Read the model definition and answer for the solid it produces. Units are mm, in the model's axes. A direction names the side the tool comes from. Coordinates: 2 decimals unless noted, no trailing zeros. Loops run counter-clockwise (first coordinate to the right, second up) from the corner with the lowest first, then second, coordinate; pieces in that order, holes last. Notation, with made-up numbers: (54.5, 63) -> (106.5, 63) arc R35 ccw to (106.5, 96) -> close; hole circle Ø10 at (1, -23). An arc over 180 degrees is marked (long way). Answer as a JSON object with one key per item and string values. Group by question number.
Q1. For faces 5 (the flat face through (-36.31, 0.99, 31.46)), 6 (the flat face through (36.307, 0.986, -31.462)), 7 (the flat face through (25.97, 0.99, -40.41)), determine the directions among +Z, -Z, +X, -X, +Y, -Y from which every point of the face is accessible in a straight line to the end or side of a thin tool.
Q2. The part is cut by section B-B on x = 29.5. Write down the section's boundary in (y, z).
Q3. Determine the mould class of faces 1 (the flat face through (36.307, 0.986, 31.462)), 2 (the flat face through (43.701, 0.986, 19.956)), 3 (the cylindrical face through (37.81, 0.99, 24.4)), 4 (the flat face through (43.701, 0.986, -19.956)) for opening direction Z: released by +Z, released by -Z, zero draft, split by the parting line, or undercut.
Q4. This flat-tipped pin is pushed along its axis until it touches: P1, Ø5, axis at x = 10.5, z = -1.5, coming from the -Y side. Where does it stop, or does it pass through?
Q5. The part is cut by section C-C on z = -26. Write down the section's boundary in (x, y).
Q6. Straight lines are drawn through the part: line 1 along Z through (x, y) = (-27, 0.9); line 2 along X through (y, z) = (0.65, 0); line 3 along Z through (x, y) = (5, 0.85). For each, find the intervals that lie inside material, in ascending order. Write a range as [from, to].
Q7. The part is cut by section A-A on z = -3. Write down the section's boundary in (x, y).
from build123d import *

# Parameters (mm, degrees)
SKETCH1_R                 = 45
BOSS_EXTRUDE1_DEPTH       = 2
BOSS_EXTRUDE2_DEPTH       = 2
CIRPATTERN1_COUNT         = 11
CIRPATTERN1_COPY_1_DEPTH  = 2
CIRPATTERN1_COPY_2_DEPTH  = 2
CIRPATTERN1_COPY_3_DEPTH  = 2
CIRPATTERN1_COPY_4_DEPTH  = 2
CIRPATTERN1_COPY_5_DEPTH  = 2
CIRPATTERN1_COPY_6_DEPTH  = 2
CIRPATTERN1_COPY_7_DEPTH  = 2
CIRPATTERN1_COPY_8_DEPTH  = 2
CIRPATTERN1_COPY_9_DEPTH  = 2
CIRPATTERN1_COPY_10_DEPTH = 2
SKETCH3_R                 = 12.5
CUT_EXTRUDE1_DEPTH        = 2


with BuildPart() as part:
    # Sketch1 → Boss-Extrude1 (new body)
    with BuildSketch(Plane(origin=(0, 0, 0), x_dir=(1, 0, 0), z_dir=(0, 1, 0))):
        Circle(SKETCH1_R)
    extrude(amount=BOSS_EXTRUDE1_DEPTH)

    # Sketch2 → Boss-Extrude2 (add)
    with BuildSketch(Plane(origin=(0, 0, 0), x_dir=(1, 0, 0), z_dir=(0, 1, 0))):
        with BuildLine():
            Line((0, 0), (-51, 0))
            ThreePointArc((-51, 0), (-50.870115566, -3.637491206), (-50.481123832, -7.256454825))
            Line((-50.481123832, -7.256454825), (0, 0))
        make_face()
    boss_extrude2 = extrude(amount=BOSS_EXTRUDE2_DEPTH)

    # Mirror1: Boss-Extrude2 across plane
    add(boss_extrude2.mirror(Plane.XY))

    # CirPattern1: Boss-Extrude2 ×11 about axis
    cirpattern1_axis = Axis((0, 0, 0), (0, 1, 0))
    for i in range(1, CIRPATTERN1_COUNT):
        add(boss_extrude2.rotate(cirpattern1_axis, i * 360 / CIRPATTERN1_COUNT))

    # CirPattern1 copy 1 sketch → CirPattern1 copy 1 (add)
    with BuildSketch(Plane(origin=(0, 0, 0), x_dir=(0.841253533, 0, -0.540640817), z_dir=(0, 1, 0))):
        with BuildLine():
            Line((0, 0), (-51, 0))
            ThreePointArc((-51, 0), (-50.870115566, 3.637491206), (-50.481123832, 7.256454825))
            Line((-50.481123832, 7.256454825), (0, 0))
        make_face()
    extrude(amount=CIRPATTERN1_COPY_1_DEPTH)

    # CirPattern1 copy 2 sketch → CirPattern1 copy 2 (add)
    with BuildSketch(Plane(origin=(0, 0, 0), x_dir=(0.415415013, 0, -0.909631995), z_dir=(0, 1, 0))):
        with BuildLine():
            Line((0, 0), (-51, 0))
            ThreePointArc((-51, 0), (-50.870115566, 3.637491206), (-50.481123832, 7.256454825))
            Line((-50.481123832, 7.256454825), (0, 0))
        make_face()
    extrude(amount=CIRPATTERN1_COPY_2_DEPTH)

    # CirPattern1 copy 3 sketch → CirPattern1 copy 3 (add)
    with BuildSketch(Plane(origin=(0, 0, 0), x_dir=(-0.142314838, 0, -0.989821442), z_dir=(0, 1, 0))):
        with BuildLine():
            Line((0, 0), (-51, 0))
            ThreePointArc((-51, 0), (-50.870115566, 3.637491206), (-50.481123832, 7.256454825))
            Line((-50.481123832, 7.256454825), (0, 0))
        make_face()
    extrude(amount=CIRPATTERN1_COPY_3_DEPTH)

    # CirPattern1 copy 4 sketch → CirPattern1 copy 4 (add)
    with BuildSketch(Plane(origin=(0, 0, 0), x_dir=(-0.654860734, 0, -0.755749574), z_dir=(0, 1, 0))):
        with BuildLine():
            Line((0, 0), (-51, 0))
            ThreePointArc((-51, 0), (-50.870115566, 3.637491206), (-50.481123832, 7.256454825))
            Line((-50.481123832, 7.256454825), (0, 0))
        make_face()
    extrude(amount=CIRPATTERN1_COPY_4_DEPTH)

    # CirPattern1 copy 5 sketch → CirPattern1 copy 5 (add)
    with BuildSketch(Plane(origin=(0, 0, 0), x_dir=(-0.959492974, 0, -0.281732557), z_dir=(0, 1, 0))):
        with BuildLine():
            Line((0, 0), (-51, 0))
            ThreePointArc((-51, 0), (-50.870115566, 3.637491206), (-50.481123832, 7.256454825))
            Line((-50.481123832, 7.256454825), (0, 0))
        make_face()
    extrude(amount=CIRPATTERN1_COPY_5_DEPTH)

    # CirPattern1 copy 6 sketch → CirPattern1 copy 6 (add)
    with BuildSketch(Plane(origin=(0, 0, 0), x_dir=(-0.959492974, 0, 0.281732557), z_dir=(0, 1, 0))):
        with BuildLine():
            Line((0, 0), (-51, 0))
            ThreePointArc((-51, 0), (-50.870115566, 3.637491206), (-50.481123832, 7.256454825))
            Line((-50.481123832, 7.256454825), (0, 0))
        make_face()
    extrude(amount=CIRPATTERN1_COPY_6_DEPTH)

    # CirPattern1 copy 7 sketch → CirPattern1 copy 7 (add)
    with BuildSketch(Plane(origin=(0, 0, 0), x_dir=(-0.654860734, 0, 0.755749574), z_dir=(0, 1, 0))):
        with BuildLine():
            Line((0, 0), (-51, 0))
            ThreePointArc((-51, 0), (-50.870115566, 3.637491206), (-50.481123832, 7.256454825))
            Line((-50.481123832, 7.256454825), (0, 0))
        make_face()
    extrude(amount=CIRPATTERN1_COPY_7_DEPTH)

    # CirPattern1 copy 8 sketch → CirPattern1 copy 8 (add)
    with BuildSketch(Plane(origin=(0, 0, 0), x_dir=(-0.142314838, 0, 0.989821442), z_dir=(0, 1, 0))):
        with BuildLine():
            Line((0, 0), (-51, 0))
            ThreePointArc((-51, 0), (-50.870115566, 3.637491206), (-50.481123832, 7.256454825))
            Line((-50.481123832, 7.256454825), (0, 0))
        make_face()
    extrude(amount=CIRPATTERN1_COPY_8_DEPTH)

    # CirPattern1 copy 9 sketch → CirPattern1 copy 9 (add)
    with BuildSketch(Plane(origin=(0, 0, 0), x_dir=(0.415415013, 0, 0.909631995), z_dir=(0, 1, 0))):
        with BuildLine():
            Line((0, 0), (-51, 0))
            ThreePointArc((-51, 0), (-50.870115566, 3.637491206), (-50.481123832, 7.256454825))
            Line((-50.481123832, 7.256454825), (0, 0))
        make_face()
    extrude(amount=CIRPATTERN1_COPY_9_DEPTH)

    # CirPattern1 copy 10 sketch → CirPattern1 copy 10 (add)
    with BuildSketch(Plane(origin=(0, 0, 0), x_dir=(0.841253533, 0, 0.540640817), z_dir=(0, 1, 0))):
        with BuildLine():
            Line((0, 0), (-51, 0))
            ThreePointArc((-51, 0), (-50.870115566, 3.637491206), (-50.481123832, 7.256454825))
            Line((-50.481123832, 7.256454825), (0, 0))
        make_face()
    extrude(amount=CIRPATTERN1_COPY_10_DEPTH)

    # Sketch3 → Cut-Extrude1 (cut)
    with BuildSketch(Plane(origin=(0, 2, 0), x_dir=(1, 0, 0), z_dir=(0, 1, 0))):
        Circle(SKETCH3_R)
    extrude(amount=-CUT_EXTRUDE1_DEPTH, mode=Mode.SUBTRACT)


solid = part.part
Final values:
{
 "1": {"face 5": "+Z, +Y, -Y", "face 6": "+X, +Y, -Y", "face 7": "-Z, +Y, -Y"},
 "2": {"outline": "(0, -41.6) -> (2, -41.6) -> (2, 41.6) -> (0, 41.6) -> close"},
 "3": {"face 1": "undercut", "face 2": "released by +Z", "face 3": "undercut", "face 4": "released by -Z"},
 "4": {"P1": "stops at y = 0"},
 "5": {"outline": "(-43.87, 0) -> (36.73, 0) -> (36.73, 2) -> (-43.87, 2) -> close"},
 "6": {"line 1": "z = [-43.27, -42.02], [-36, 36], [42.02, 43.27]", "line 2": "x = [-51, -12.5], [12.5, 45]", "line 3": "z = [-50.75, -11.46], [11.46, 50.75]"},
 "7": {"outline": "(-50.91, 0) -> (-12.13, 0) -> (-12.13, 2) -> (-50.91, 2) -> close; (12.13, 0) -> (44.9, 0) -> (44.9, 2) -> (12.13, 2) -> close"}
}
